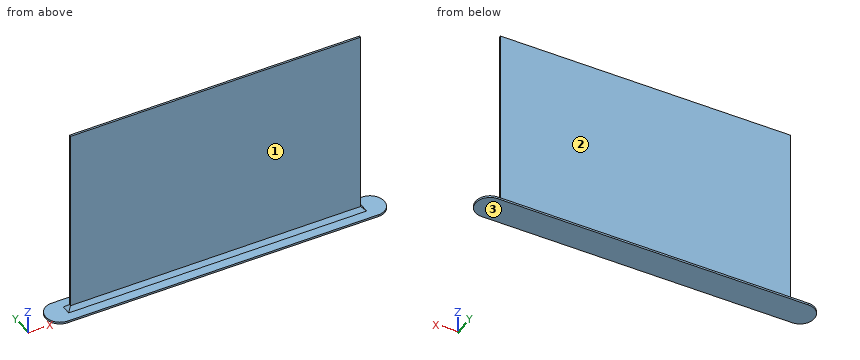
from build123d import *

# Parameters (mm, degrees)
F0_W     = 150
F0_H     = 1
F1_DEPTH = 100
F2_W     = 175
F2_H     = 15
F3_DEPTH = 1
F4_R     = 7.242641
F5_SIZE  = 2


with BuildPart() as f1:
    # F0 (on Top) → F1 (new body)
    with BuildSketch(Plane.XY):
        Rectangle(F0_W, F0_H)
    extrude(amount=F1_DEPTH)

    # F2 (on Top) → F3 (join)
    with BuildSketch(Plane.XY):
        Rectangle(F2_W, F2_H)
    extrude(amount=F3_DEPTH)

    # F4
    f4_edges = [f1.edges().sort_by_distance(p)[0] for p in [
        (-87.5, -7.5, 0.5),
        (-87.5, 7.5, 0.5),
        (87.5, -7.5, 0.5),
        (87.5, 7.5, 0.5),
    ]]
    fillet(f4_edges, radius=F4_R)

    # F5
    f5_edges = [f1.edges().sort_by_distance(p)[0] for p in [
        (0, 0.5, 1),
        (75, 0, 1),
        (0, -0.5, 1),
        (-75, 0, 1),
    ]]
    chamfer(f5_edges, length=F5_SIZE)


solid = f1.part
Could you check a few things on this model? Use its own coordinates, in mm. Face numbers are marked on the shaded views. A direction names the side the tool comes from. Give positions to 0.01 mm unless a question says otherwise; leave off trailing zeros. Order: outer loops, then holes, each group sorted by start corner. A loop starts at its lowest first (then second) coordinate and runs counter-clockwise, first axis right, second up. Notation, with made-up numbers: (30, -31.75) - (72, -31.75) arc R28 ccw to (72, -10.75) - close; hole circle Ø4 at (58, -26). An arc over 180 degrees is marked (long way). One line per item, written item: value. Start each with the question number.
1. Imagine slicing it at C-C on y = 5.5. List the corners of the cut face in (x, z) for me, plus the area to 3 significant figures.
2. Imagine slicing it at A-A on x = -29. List the corners of the cut face in (y, z) for me.
3. For the marked faces 1, 2 and 3, which set-ups out of +Z, -Z, +X, -X, +Y, -Y let a thin tool reach every point of the face, with its end or its side?
4. If I drill on probe 1 along Y at (x, z) = (-64, 12); probe 2 along Z at (x, y) = (51, 4.25); probe 3 along X at (y, z) = (0, 71), over which ranges is the centre line in solid material (lowest first)?
5. Imagine slicing it at B-B on z = 63.5. List the corners of the cut face in (x, y) for me.
6. For P1, Ø1.5, axis at x = 18.5, z = 63, coming from the -Y side; P2, Ø6, axis at x = 52.5, y = 4.5, coming from the +Z side; P3, Ø6, axis at x = -34, z = 70, coming from the +Y side, each with a flat end and sliding along its axis, tell me the tip position at first contact or that it passes through.
Values:
1. outline: (-85.25, 0) - (85.25, 0) - (85.25, 1) - (-85.25, 1) - close
1. area: 171 mm²
2. outline: (-7.5, 0) - (7.5, 0) - (7.5, 1) - (2.5, 1) - (0.5, 3) - (0.5, 100) - (-0.5, 100) - (-0.5, 3) - (-2.5, 1) - (-7.5, 1) - close
3. face 1: +Z, +X, -X, -Y
3. face 2: +Z, +X, -X, +Y
3. face 3: -Z, +X, -X, +Y, -Y
4. probe 1: -0.5 to 0.5
4. probe 2: 0 to 1
4. probe 3: -75 to 75
5. outline: (-75, -0.5) - (75, -0.5) - (75, 0.5) - (-75, 0.5) - close
6. P1: y = -0.5
6. P2: z = 2
6. P3: y = 0.5
